The listing builds one solid part. Answer for the finished solid, in the listing's coordinates (mm). A direction names the side the tool comes from. Give positions to 0.01 mm unless a question says otherwise; leave off trailing zeros. Order: outer loops, then holes, each group sorted by start corner. A loop starts at its lowest first (then second) coordinate and runs counter-clockwise, first axis right, second up. Notation, with made-up numbers: (11.25, 71) - (47.25, 71) arc R14 ccw to (47.25, 75) - close; hole circle Ø8 at (39, -32.75). An arc over 180 degrees is marked (long way). Answer in a Markdown table with one row per item.
from build123d import *

# Parameters (mm, degrees)
BOSS_EXTRUDE1_DEPTH = 90
SKETCH2_R           = 5
CUT_EXTRUDE1_DEPTH  = 90


with BuildPart() as part:
    # Sketch1 → Boss-Extrude1 (new body)
    with BuildSketch(Plane.XY):
        Polygon((-51.967349513, 26.424347916), (129.032650487, 26.424347916), (129.032650487, -18.575652084), (159.032650487, -18.575652084), (159.032650487, -21.575652084), (129.032650487, -21.575652084), (126.032650487, -21.575652084), (126.032650487, 23.424347916), (-48.967349513, 23.424347916), (-48.967349513, -21.575652084), (-51.967349513, -21.575652084), (-81.967349513, -21.575652084), (-81.967349513, -18.575652084), (-51.967349513, -18.575652084), align=None)
    extrude(amount=BOSS_EXTRUDE1_DEPTH)

    # Sketch2 → Cut-Extrude1 (cut)
    with BuildSketch(Plane(origin=(0, -18.575652084, 0), x_dir=(1, 0, 0), z_dir=(0, 1, 0))):
        with Locations((144.032650487, -22.5)):
            Circle(SKETCH2_R)
        with Locations((144.032650487, -67.5)):
            Circle(SKETCH2_R)
        with Locations((-66.967349513, -67.5)):
            Circle(SKETCH2_R)
        with Locations((-66.967349513, -22.5)):
            Circle(SKETCH2_R)
    extrude(amount=-CUT_EXTRUDE1_DEPTH, mode=Mode.SUBTRACT)


solid = part.part
Item 1: Find section B-B on y = 16. Write down the section's boundary in (x, z), then the cut area to 3 significant figures.
Answer block:
| item | result |
|---|---|
| outline | (-51.97, 0) - (-48.97, 0) - (-48.97, 90) - (-51.97, 90) - close; (126.03, 0) - (129.03, 0) - (129.03, 90) - (126.03, 90) - close |
| area | 540 mm² |
Item 2: Consider line 1 (X direction, y = -20, z = 67); line 2 (X direction, y = -19.85, z = 67.5); line 3 (X direction, y = 17, z = 28). Determine where each line is inside the solid, lowest interval first.
Answer block:
| item | result |
|---|---|
| line 1 | -81.97 to -71.94, -61.99 to -48.97, 126.03 to 139.06, 149.01 to 159.03 |
| line 2 | -81.97 to -71.97, -61.97 to -48.97, 126.03 to 139.03, 149.03 to 159.03 |
| line 3 | -51.97 to -48.97, 126.03 to 129.03 |
Item 3: Determine the mould class of faces 4 (the face through (129.033, 4, 44)), 5 (the face through (148.802, -20.055, 65.998)), 6 (the face through (39, 26, 0)) for opening direction X: pulls with the +X half, pulls with the -X half, needs draft (parallel to the pull), parting line crosses it, or undercut.
Answer block:
| item | result |
|---|---|
| face 4 | pulls with the +X half |
| face 5 | undercut |
| face 6 | needs draft |
Item 4: Which of the six approach directions +Z, -Z, +X, -X, +Y, -Y give full straight-line access (tool end or side, diameter ignored) to faces 1 (the face through (144, -18.576, 44)), 2 (the face through (40, 23.424, 44)), 3 (the face through (-51.967, 4, 44))?
Answer block:
| item | result |
|---|---|
| face 1 | +Z, -Z, +X, +Y |
| face 2 | +Z, -Z, -Y |
| face 3 | +Z, -Z, -X, +Y |
Item 5: Find section A-A on z = 67.5. Write down the section's boundary in (x, y).
Answer block:
| item | result |
|---|---|
| outline | (-81.97, -21.58) - (-71.97, -21.58) - (-71.97, -18.58) - (-81.97, -18.58) - close; (-61.97, -21.58) - (-48.97, -21.58) - (-48.97, 23.42) - (126.03, 23.42) - (126.03, -21.58) - (139.03, -21.58) - (139.03, -18.58) - (129.03, -18.58) - (129.03, 26.42) - (-51.97, 26.42) - (-51.97, -18.58) - (-61.97, -18.58) - close; (149.03, -21.58) - (159.03, -21.58) - (159.03, -18.58) - (149.03, -18.58) - close |
Item 6: Find section C-C on x = 6.5. Write down the section's boundary in (y, z).
Answer block:
| item | result |
|---|---|
| outline | (23.42, 0) - (26.42, 0) - (26.42, 90) - (23.42, 90) - close |
Item 7: Each of these flat-tipped pins is pushed along its axis until it touches: P1, Ø15, axis at x = -71.5, z = 59.5, coming from the +Y side; P2, Ø4, axis at x = 42.5, z = 67.5, coming from the -Y side; P3, Ø13.5, axis at y = -7.5, z = 31.5, coming from the -X side; P4, Ø13, axis at x = 144.03, z = 22.5, coming from the -Y side. Where does it stop, or does it pass through?
Answer block:
| item | result |
|---|---|
| P1 | y = -18.58 |
| P2 | y = 23.42 |
| P3 | x = -51.97 |
| P4 | y = -21.58 |
